Build history of the part. All positions in model axes, mm. A direction names the side the tool comes from. Round coordinates to 2 decimals unless told otherwise and drop trailing zeros. Write each loop counter-clockwise with the first axis right and the second up, starting at its lowest first coordinate (ties: lowest second). Pieces come first, ordered by that corner, then holes. Notation, with made-up numbers: M -24,2.25 L 32,2.25 A27 cw 32,38.25 Z; hole C 28,-14.75 d1. An arc over 180 degrees is marked long. Write item = value, one per line.
Autodesk Fusion 360 part; units mm, degrees
sketch "Sketch1" plane through (0, 0, 0) normal (0, 0, 1) x (1, 0, 0)
  circle A0 centre (0, 0) radius 21.3
  line L0 (0, 0) -> (-15.0614, -15.0614)
  line L1 (0, 0) -> (21.3, 0) construction
  line L2 (-15.0614, -15.0614) -> (-23.0517, -23.0517)
  circle A1 centre (-23.0517, -23.0517) radius 11
  line L3 (0, 0) -> (15.0614, -15.0614)
  line L4 (15.0614, -15.0614) -> (23.0517, -23.0517)
  circle A2 centre (23.0517, -23.0517) radius 11
  circle A3 centre (-23.0517, 23.0517) radius 11
  circle A4 centre (23.0517, 23.0517) radius 11
  line L5 (-23.0517, 23.0517) -> (-35.0517, 23.0517)
  line L6 (-35.0517, 23.0517) -> (-35.0517, -36.9483)
  line L7 (23.0517, 23.0517) -> (35.0517, 23.0517)
  line L8 (35.0517, 23.0517) -> (35.0517, -36.9483)
  line L9 (35.0517, -36.9483) -> (-35.0517, -36.9483)
  line L10 (-23.0517, 23.0517) -> (23.0517, 23.0517)
  circle A5 centre (-23.0517, 23.0517) radius 4
  circle A6 centre (23.0517, 23.0517) radius 4
  circle A7 centre (23.0517, -23.0517) radius 4
  circle A8 centre (-23.0517, -23.0517) radius 4
  line L11 (-35.0517, 23.0517) -> (-35.0517, 24)
  line L12 (-35.0517, 24) -> (-35.0517, 28.0517)
  line L13 (-35.0517, 28.0517) -> (35.0082, 28.0517)
  line L14 (35.0082, 28.0517) -> (35.0517, 23.0517)
  line L15 (-23.0517, -23.0517) -> (-18.1019, -18.1019)
  line L16 (-23.0517, 23.0517) -> (-18.1019, 18.1019)
  line L17 (23.0517, 23.0517) -> (18.1019, 18.1019)
  line L18 (23.0517, 23.0517) -> (30.0517, 23.0517) construction
  line L19 (23.0517, -23.0517) -> (18.1019, -18.1019)
  arc A9 (18.1019, 18.1019) -> (-18.1019, 18.1019) centre (0, -12.5239) ccw
  line L20 (0, 0) -> (-21.3, 0)
  line L21 (-21.3, 0) -> (-22.3, 0)
  arc A10 (-18.1019, 18.1019) -> (-18.1019, -18.1019) centre (18.8265, 0) ccw
  line L22 (0, 0) -> (0, 5) construction
  arc A11 (18.1019, -18.1019) -> (18.1019, 18.1019) centre (-18.8265, 0) ccw
  line L23 (0, 0) -> (0, -21.3)
  line L24 (0, -21.3) -> (0, -22.3)
  arc A12 (-18.1019, -18.1019) -> (18.1019, -18.1019) centre (0, 18.8265) ccw
  line L25 (0, 0) -> (0, -21.3)
  line L26 (0, -21.3) -> (0, -29.3)
  line L27 (-21.3, 0) -> (-29.3, 0)
  line L28 (21.3, 0) -> (29.3, 0)
  circle A13 centre (29.3, 0) radius 1.5
  circle A14 centre (0, -29.3) radius 1.5
  circle A15 centre (-29.3, 0) radius 1.5
  dimension "d1" = 42.6
  dimension "d2" = 135
  dimension "d3" = 11.3
  dimension "d4" = 22
  dimension "d5" = 11.3
  dimension "d6" = 22
  dimension "d7" = 12
  dimension "d8" = 60
  dimension "d9" = 12
  dimension "d10" = 60
  dimension "d11" = 8
  dimension "d12" = 8
  dimension "d13" = 8
  dimension "d14" = 8
  dimension "d15" = 5
  dimension "d16" = 7
  dimension "d17" = 7
  dimension "d18" = 135
  dimension "d19" = 7
  dimension "d20" = 7
  dimension "d25" = 1
  dimension "d26" = 1
  dimension "d27" = 8
  dimension "d28" = 8
  dimension "d29" = 8
  dimension "d30" = 3
  dimension "d31" = 3
  dimension "d32" = 3
extrude "Extrude1" add sketch "Sketch1" along normal blind 5 contours A1 A2 A3 A4 L5 L6 L7 L8 L9 A10 A11 A12 | A2 A11 A12 | A4 L7 A6 L17 A11 | A3 L5 A5 L16 A10 | A1 A10 A12 | A4 L10 A9 | A4 L10 A6 L17 A9 | A4 L7 L10 A6 L13 | A4 L7 L13 L14 | A3 L5 L11 L12 L13 | A3 L5 L10 A5 L13 | A3 L10 A5 L16 A9 | A3 L10 A9 | A3 A4 L10 L13
1. Mould opens along Y. For faces 1 (the face through (0, -36.948, 2)), 2 (the face through (-26.226, 25.486, 2.465)), 3 (the face through (22.3, 0.3, 2.5)), 4 (the face through (35.052, -7, 2)) say: pulls with the +Y half, pulls with the -Y half, needs draft (parallel to the pull), parting line crosses it, or undercut.
Responses:
face_1 = pulls with the -Y half
face_2 = undercut
face_3 = undercut
face_4 = needs draft
2. Band-saw the part on D-D (y = -29.3). List the corners of the cut face in (x, z), plus the area to 3 significant figures.
Responses:
outline = M -35.05,0 L -1.5,0 L -1.5,5 L -35.05,5 Z; M 1.5,0 L 35.05,0 L 35.05,5 L 1.5,5 Z
area = 336 mm²
3. Band-saw the part on A-A (x = -29.3). List the corners of the cut face in (y, z).
Responses:
outline = M -36.95,0 L -1.5,0 L -1.5,5 L -36.95,5 Z; M 1.5,0 L 28.05,0 L 28.05,5 L 1.5,5 Z
4. Band-saw the part on C-C (x = 0). List the corners of the cut face in (y, z), plus the area to 3 significant figures.
Responses:
outline = M -36.95,0 L -30.8,0 L -30.8,5 L -36.95,5 Z; M -27.8,0 L -22.3,0 L -22.3,5 L -27.8,5 Z; M 23.05,0 L 28.05,0 L 28.05,5 L 23.05,5 Z
area = 83.2 mm²
5. Tool access for faces 5 (the face through (0.3, -22.3, 2.5)), 6 (the face through (-1, 28.052, 2)): list every direction of +Z, -Z, +X, -X, +Y, -Y with a clear straight run to the whole face (end or side of a thin tool).
Responses:
face_5 = +Z, -Z
face_6 = +Z, -Z, +X, -X, +Y
6. Flat gauge pin, fed straight in: pin 1 (6.5 mm diameter, centred on x = 23.05, y = 23.05, fed in from -Z). Where does the tip first touch, or does it go through?
Responses:
pin_1 = through
7. Band-saw the part on B-B (y = 0). List the corners of the cut face in (x, z).
Responses:
outline = M -35.05,0 L -30.8,0 L -30.8,5 L -35.05,5 Z; M -27.8,0 L -22.3,0 L -22.3,5 L -27.8,5 Z; M 22.3,0 L 27.8,0 L 27.8,5 L 22.3,5 Z; M 30.8,0 L 35.05,0 L 35.05,5 L 30.8,5 Z
8. Probe probe 1 along Y at (x, z) = (0, 1.15); probe 2 along X at (y, z) = (25.5, 1.65); probe 3 along X at (y, z) = (-22.5, 2). List the from-to ranges inside material, lowest first.
Responses:
probe_1 = -36.95 to -30.8, -27.8 to -22.3, 23.05 to 28.05
probe_2 = -35.05 to -26.21, -19.89 to 19.89, 26.21 to 35.03
probe_3 = -35.05 to -27.01, -19.09 to 19.09, 27.01 to 35.05
